Verification items for the finished model (mm, model axes). A direction names the side the tool comes from. Round coordinates to 2 decimals unless told otherwise and drop trailing zeros. Order: outer loops, then holes, each group sorted by start corner. A loop starts at its lowest first (then second) coordinate and runs counter-clockwise, first axis right, second up. Notation, with made-up numbers: (41, 26.5) -> (92, 26.5) arc R14 cw to (92, 35.5) -> close; hole circle Ø10 at (56, -38). An arc over 180 degrees is marked (long way). Return JSON: item names as keys, results as strings. Group by question number.
Item 1: Draft check along X on faces 3 (the cylindrical face through (-0.69, -3.1, 19.98)), 4 (the flat face through (4, 0, 18.542)), 5 (the cylindrical face through (-0.69, -0.13, 6.17)). Enter one of: pulls with the +X half, pulls with the -X half, needs draft (parallel to the pull), parting line crosses it, or undercut.
Item 2: Sectioned sample at B-B on y = -2. Record the cut outline in (x, z) (3 decimals).
Item 3: Depth check by flat-ended pin: pin 1 Ø4 at (y, z) = (-5, 5.5) entering from +X; pin 2 Ø8 at (y, z) = (5, 1.5) entering from +X; pin 3 Ø5.5 at (x, z) = (0, 9.271) entering from -Y; pin 4 Ø1 at (x, y) = (5.5, 2) entering from +Z. Enter the tip coordinate at first touch or a pass-through.
Item 4: Scan lines: probe 1 along Z at (x, y) = (0, 1.75); probe 2 along Z at (x, y) = (0, -4.5); probe 3 along X at (y, z) = (-7, 8). Record each from-to range of solid material in increasing order. Write a range as from..to.
Item 5: Access from +Z, -Z, +X, -X, +Y, -Y to the whole of each face (thin tool, end or side, straight path). Record for faces 1 (the cylindrical face through (-0.69, 3.1, -1.44)), 2 (the flat face through (0, 0, 21.463)).
Item 6: Sectioned sample at D-D on x = 2.5. Record the cut outline in (y, z), plus the area to 3 significant figures.
Item 7: Sectioned sample at A-A on x = 0. Record the cut outline in (y, z) (3 decimals), plus the area to 3 significant figures.
Item 8: Sectioned sample at C-C on z = 17.75. Record the cut outline in (x, y) (3 decimals).
```python
from build123d import *

# Parameters (mm, degrees)
F0_R          = 9.525
F1_DEPTH      = 18.542
F2_R          = 3.175
F3_DEPTH      = 2.921
F4_R          = 3.175
F5_DEPTH      = 2.921
F6_R          = 3.175
F7_DEPTH      = 25.4
F7_DEPTH_BACK = 25.4


with BuildPart() as f1:
    # F0 (on Top) → F1 (new body)
    with BuildSketch(Plane.XY):
        Circle(F0_R)
    extrude(amount=F1_DEPTH)

    # F2 (on face) → F3 (join)
    with BuildSketch(Plane.XY.offset(18.542)):
        Circle(F2_R)
    extrude(amount=F3_DEPTH)

    # F4 (on face) → F5 (join)
    with BuildSketch(Plane(origin=(0, 0, 0), x_dir=(1, 0, 0), z_dir=(0, 0, -1))):
        Circle(F4_R)
    extrude(amount=F5_DEPTH)

    # F6 (on Front) → F7 (cut, two sides)
    with BuildSketch(Plane.XZ) as f7_sk:
        with Locations((0, 9.271)):
            Circle(F6_R)
    extrude(amount=-F7_DEPTH, mode=Mode.SUBTRACT)
    extrude(f7_sk.sketch, amount=F7_DEPTH_BACK, mode=Mode.SUBTRACT)


solid = f1.part
```
Recorded:
{
 "1": {"face 3": "parting line crosses it", "face 4": "needs draft", "face 5": "undercut"},
 "2": {"outline": "(-9.313, 0) -> (-2.466, 0) -> (-2.466, -2.921) -> (2.466, -2.921) -> (2.466, 0) -> (9.313, 0) -> (9.313, 18.542) -> (2.466, 18.542) -> (2.466, 21.463) -> (-2.466, 21.463) -> (-2.466, 18.542) -> (-9.313, 18.542) -> close; hole circle Ø6.35 at (0, 9.271)"},
 "3": {"pin 1": "x = 9.04", "pin 2": "x = 9.47", "pin 3": "through", "pin 4": "z = 18.54"},
 "4": {"probe 1": "-2.92..6.1, 12.45..21.46", "probe 2": "0..6.1, 12.45..18.54", "probe 3": "-6.46..-2.91, 2.91..6.46"},
 "5": {"face 1": "-Z", "face 2": "+Z, +X, -X, +Y, -Y"},
 "6": {"outline": "(-9.19, 0) -> (-1.96, 0) -> (-1.96, -2.92) -> (1.96, -2.92) -> (1.96, 0) -> (9.19, 0) -> (9.19, 7.31) -> (-9.19, 7.31) -> close; (-9.19, 11.23) -> (9.19, 11.23) -> (9.19, 18.54) -> (1.96, 18.54) -> (1.96, 21.46) -> (-1.96, 21.46) -> (-1.96, 18.54) -> (-9.19, 18.54) -> close", "area": "292 mm²"},
 "7": {"outline": "(-9.525, 0) -> (-3.175, 0) -> (-3.175, -2.921) -> (3.175, -2.921) -> (3.175, 0) -> (9.525, 0) -> (9.525, 6.096) -> (-9.525, 6.096) -> close; (-9.525, 12.446) -> (9.525, 12.446) -> (9.525, 18.542) -> (3.175, 18.542) -> (3.175, 21.463) -> (-3.175, 21.463) -> (-3.175, 18.542) -> (-9.525, 18.542) -> close", "area": "269 mm²"},
 "8": {"outline": "circle Ø19.05 at (0, 0)"}
}
